Model file for the job. Use its own axes, mm. Face numbers are marked on the shaded views. A direction names the side the tool comes from. Coordinates: 2 decimals unless noted, no trailing zeros. Write each loop counter-clockwise with the first axis right and the second up, starting at its lowest first coordinate (ties: lowest second). Pieces come first, ordered by that corner, then holes. Notation, with made-up numbers: (-17, 51) - (6, 51) arc R27 cw to (6, 83) - close; hole circle Ø10 at (-5.5, 44.25). An arc over 180 degrees is marked (long way). Put each result on its own line as item: value. Start each with the question number.
1. Which spindle directions (+Z, -Z, +X, -X, +Y, -Y) get a long thin tool onto all of the face, cutting with end or side? Do the marked faces 1, 2 and 3. Say none if no direction does.
2. Saw through at A-A, the plane y = -9. Write the cut outline in (x, z).
3. Saw through at B-B, the plane z = 0. Write the cut outline in (x, y), plus the area to 3 significant figures.
4. Saw through at D-D, the plane z = -5.25. Write the cut outline in (x, y), plus the area to 3 significant figures.
5. Drill centre lines: L1, parallel to Z at x = -5, y = 0; L2, parallel to Z at x = -1.8, y = -8; L3, parallel to Y at x = -2.25, z = -7.25. Where is each one in solid material? Low to high. Write a range as from..to.
6. Drop flat-ended pins along their axis: P1, Ø2, axis at x = -3, y = -7, coming from the +Z side; P2, Ø1, axis at x = -2, z = -4.5, coming from the -Y side; P3, Ø1.5, axis at x = -3, y = -7.5, coming from the -Z side; P4, Ø4, axis at y = -0.5, z = 6.5, coming from the -X side. Give the stop position or say it passes through.
7. Saw through at C-C, the plane y = 0.25. Write the cut outline in (x, z), plus the area to 3 significant figures.
8. Pull direction Z, two halves, no side cores. Call the marked faces 4, 5 and 6: released by +Z, released by -Z, zero draft, split by the parting line, or undercut.
```python
from build123d import *

# Parameters (mm, degrees)
SKETCH2_R          = 1.6256
CUT_EXTRUDE1_DEPTH = 3.556
CIRPATTERN1_COUNT  = 4
CUT_EXTRUDE2_DEPTH = 3.556
SKETCH4_R          = 4.99999
CUT_EXTRUDE3_DEPTH = 10
CUT_EXTRUDE4_DEPTH = 3.556
SKETCH6_R          = 5.08
CUT_EXTRUDE5_DEPTH = 1.5824
CUT_EXTRUDE6_DEPTH = 4.556
FILLET1_R          = 0.635


with BuildPart() as part:
    # Sketch1 → Revolve1 (revolve)
    with BuildSketch(Plane.XY):
        Polygon((-15.1384, 4.99999), (-5.1384, 4.99999), (-5.1384, 11), (-1.5824, 11), (-1.5824, 5.08), (0, 5.08), (0, 4), (-15.1384, 4), align=None)
    revolve(axis=Axis((0, 0, 0), (-1, 0, 0)))

    # Sketch2 → Cut-Extrude1 (cut)
    with BuildSketch(Plane(origin=(-1.5824, 0, 0), x_dir=(0, 0, -1), z_dir=(1, 0, 0))):
        with Locations((0, 7.97105)):
            Circle(SKETCH2_R)
    cut_extrude1 = extrude(amount=-CUT_EXTRUDE1_DEPTH, mode=Mode.SUBTRACT)

    # CirPattern1: Cut-Extrude1 ×4 about axis
    cirpattern1_axis = Axis((0, 0, 0), (1, 0, 0))
    for i in range(1, CIRPATTERN1_COUNT):
        add(cut_extrude1.rotate(cirpattern1_axis, i * 360 / CIRPATTERN1_COUNT), mode=Mode.SUBTRACT)

    # Sketch3 → Cut-Extrude2 (cut)
    with BuildSketch(Plane(origin=(-1.5824, 0, 0), x_dir=(0, 0, -1), z_dir=(1, 0, 0))):
        with BuildLine():
            Line((-4.215969639, 10.16), (4.215969639, 10.16))
            ThreePointArc((4.215969639, 10.16), (0, 11), (-4.215969639, 10.16))
        make_face()
    extrude(amount=-CUT_EXTRUDE2_DEPTH, mode=Mode.SUBTRACT)

    # Sketch4 → Cut-Extrude3 (cut)
    with BuildSketch(Plane.ZY.offset(15.1384)):
        Circle(SKETCH4_R)
    extrude(amount=-CUT_EXTRUDE3_DEPTH, mode=Mode.SUBTRACT)

    # Sketch5 → Cut-Extrude4 (cut)
    with BuildSketch(Plane.ZY.offset(5.1384)):
        with BuildLine():
            ThreePointArc((-4, 0), (-7.5, 3.5), (-11, 0))
            ThreePointArc((-11, 0), (0, 11), (11, 0))
            ThreePointArc((11, 0), (7.5, 3.5), (4, 0))
            ThreePointArc((4, 0), (0, 4), (-4, 0))
        make_face()
    extrude(amount=-CUT_EXTRUDE4_DEPTH, mode=Mode.SUBTRACT)

    # Sketch6 → Cut-Extrude5 (cut)
    with BuildSketch(Plane(origin=(0, 0, 0), x_dir=(0, 0, -1), z_dir=(1, 0, 0))):
        Circle(SKETCH6_R)
    extrude(amount=-CUT_EXTRUDE5_DEPTH, mode=Mode.SUBTRACT)

    # Sketch7 → Cut-Extrude6 (cut, through all)
    with BuildSketch(Plane.ZY.offset(5.1384)):
        with BuildLine():
            Line((-7.97105, 1.6256), (-6.133690597, 1.6256))
            ThreePointArc((-6.133690597, 1.6256), (0, 6.34545), (6.133690597, 1.6256))
            Line((6.133690597, 1.6256), (7.97105, 1.6256))
            ThreePointArc((7.97105, 1.6256), (6.34545, 0), (7.97105, -1.6256))
            Line((7.97105, -1.6256), (6.133690597, -1.6256))
            ThreePointArc((6.133690597, -1.6256), (4.486910725, -4.486910725), (1.6256, -6.133690597))
            Line((1.6256, -6.133690597), (1.6256, -7.97105))
            ThreePointArc((1.6256, -7.97105), (0, -6.34545), (-1.6256, -7.97105))
            Line((-1.6256, -7.97105), (-1.6256, -6.133690597))
            ThreePointArc((-1.6256, -6.133690597), (-4.486910725, -4.486910725), (-6.133690597, -1.6256))
            Line((-6.133690597, -1.6256), (-7.97105, -1.6256))
            ThreePointArc((-7.97105, -1.6256), (-6.34545, 0), (-7.97105, 1.6256))
        make_face()
    extrude(amount=-CUT_EXTRUDE6_DEPTH, mode=Mode.SUBTRACT)

    # Fillet1
    fillet1_edges = [part.edges().sort_by_distance(p)[0] for p in [
        (-3.3604, 2.95072108, 5.617649047),
        (-3.3604, 1.6256, -6.133690597),
        (-3.3604, 1.6256, 6.133690597),
        (-3.3604, 2.95072108, -5.617649047),
    ]]
    fillet(fillet1_edges, radius=FILLET1_R)


solid = part.part
```
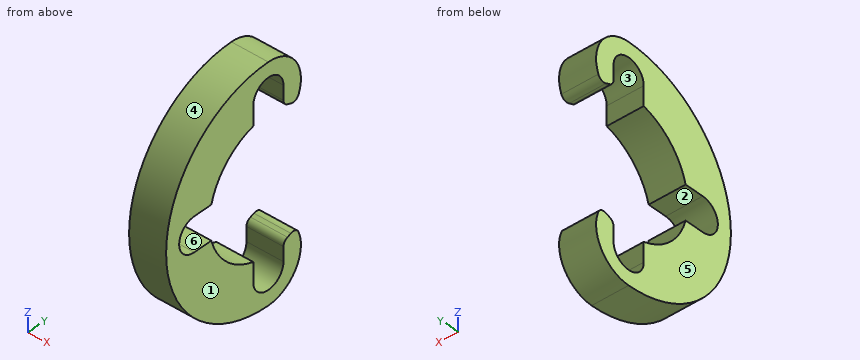
Final values:
1. face 1: +Z, -Z, +X, +Y, -Y
1. face 2: +X, -X, +Y
1. face 3: +X, -X
2. outline: (-5.14, -6.32) - (-1.58, -6.32) - (-1.58, -1.26) - (-5.14, -1.26) - close; (-5.14, 1.26) - (-1.58, 1.26) - (-1.58, 6.32) - (-5.14, 6.32) - close
3. outline: (-5.14, -11) - (-1.58, -11) - (-1.58, -9.6) - (-5.14, -9.6) - close
3. area: 4.99 mm²
4. outline: (-5.14, -9.67) - (-1.58, -9.67) - (-1.58, -3.56) - (-5.14, -3.56) - close
4. area: 21.7 mm²
5. L1: z = -11..-9.6, 9.6..11
5. L2: z = -7.55..-1.63, 1.63..7.55
5. L3: y = -8.27..-1.63, 1.63..3.49
6. P1: stops at z = 9.22
6. P2: stops at y = -10.25
6. P3: stops at z = -8.69
6. P4: stops at x = -5.14
7. outline: (-5.14, -10.99) - (-1.58, -10.99) - (-1.58, -9.58) - (-5.14, -9.58) - close; (-5.14, 9.58) - (-1.58, 9.58) - (-1.58, 10.99) - (-5.14, 10.99) - close
7. area: 10.1 mm²
8. face 4: split by the parting line
8. face 5: zero draft
8. face 6: undercut
